from build123d import *

# Parameters (mm, degrees)
SKETCH_R        = 7.5
PAD_DEPTH       = 92
POCKET_DEPTH    = 3
POCKET001_DEPTH = 9.701
POCKET002_DEPTH = 3.7


with BuildPart() as part:
    # Sketch → Pad (new body)
    with BuildSketch(Plane.YZ):
        with BuildLine():
            Line((-25.389858, -4.25), (17.999978, -4.25))
            ThreePointArc((17.999978, -4.25), (22.123115, 11.683029), (10.788897, -0.25))
            Line((-10.788897, -0.25), (10.788897, -0.25))
            ThreePointArc((-10.788897, -0.25), (-13.649082, 11.552021), (-25.389858, 8.45))
            Line((-43.389858, 8.45), (-25.389858, 8.45))
            Line((-43.389858, -4.25), (-43.389858, 8.45))
            Line((-25.389858, -4.25), (-43.389858, -4.25))
        make_face()
        with Locations((-18, 4.25)):
            Circle(SKETCH_R, mode=Mode.SUBTRACT)
        with Locations((18, 4.25)):
            Circle(SKETCH_R, mode=Mode.SUBTRACT)
    extrude(amount=PAD_DEPTH)

    # Sketch001 → Pocket (cut)
    with BuildSketch(Plane(origin=(0, 0, 8.45), x_dir=(0, -1, 0), z_dir=(0, 0, 1))):
        with BuildLine():
            ThreePointArc((43.35, 24), (35.35, 16), (43.35, 8))
            Line((50.35, 8), (43.35, 8))
            Line((50.35, 24), (50.35, 8))
            Line((43.35, 24), (50.35, 24))
        make_face()
        with BuildLine():
            ThreePointArc((43.349998, 84), (35.35, 76), (43.349998, 68))
            Line((59.835098, 68), (43.349998, 68))
            Line((59.835098, 84), (59.835098, 68))
            Line((43.349998, 84), (59.835098, 84))
        make_face()
    extrude(amount=-POCKET_DEPTH, mode=Mode.SUBTRACT)

    # Sketch002 → Pocket001 (cut, through all)
    with BuildSketch(Plane(origin=(0, 0, 5.45), x_dir=(0, -1, 0), z_dir=(0, 0, 1))):
        with BuildLine():
            ThreePointArc((43.35, 22), (37.35, 16), (43.35, 10))
            Line((53.35, 10), (43.35, 10))
            Line((53.35, 22), (53.35, 10))
            Line((43.35, 22), (53.35, 22))
        make_face()
        with BuildLine():
            ThreePointArc((43.35, 82), (37.35, 76.000014), (43.349973, 70))
            Line((53.35, 70), (43.349973, 70))
            Line((53.35, 82), (53.35, 70))
            Line((43.35, 82), (53.35, 82))
        make_face()
    extrude(amount=-POCKET001_DEPTH, mode=Mode.SUBTRACT)

    # Sketch003 → Pocket002 (cut)
    with BuildSketch(Plane.YX.offset(4.25)):
        with BuildLine():
            ThreePointArc((-43.349996, 68), (-35.35, 76.000002), (-43.35, 84))
            Line((-43.35, 84), (-53.35, 84))
            Line((-53.35, 84), (-53.35, 68))
            Line((-53.35, 68), (-43.349996, 68))
        make_face()
        with BuildLine():
            ThreePointArc((-43.35, 8), (-35.35, 16), (-43.35, 24))
            Line((-43.35, 24), (-53.350004, 24))
            Line((-53.350004, 24), (-53.350004, 8))
            Line((-53.350004, 8), (-43.35, 8))
        make_face()
    extrude(amount=-POCKET002_DEPTH, mode=Mode.SUBTRACT)


solid = part.part
Read the model definition and answer for the solid it produces. Units are mm, in the model's axes. A direction names the side the tool comes from. Round coordinates to 2 decimals unless told otherwise and drop trailing zeros. Loops run counter-clockwise (first coordinate to the right, second up) from the corner with the lowest first, then second, coordinate; pieces in that order, holes last.
Q1. Each of these flat-tipped pins is pushed along its axis until it touches: pin 1 (6.5 mm diameter, centred on x = 59, y = -4.5, fed in from +Z); pin 2 (4 mm diameter, centred on x = 80, y = -39.5, fed in from -Z); pin 3 (10 mm diameter, centred on y = 9.5, z = 10.5, fed in from -X); pin 4 (5.5 mm diameter, centred on x = 69, y = -35.5, fed in from +Z). Where does it stop, or does it pass through?
Q2. Section D-D on x = 16 is taken. Write down the section's boundary in (y, z), and give its area (3 significant figures).
Q3. Consider probe 1 along Y at (x, z) = (48, 4); probe 2 along Z at (x, y) = (72, -18); probe 3 along Y at (x, z) = (19, 6.5). Determine where each line is inside the solid, lowest interval first.
Q4. Which of the six approach directions +Z, -Z, +X, -X, +Y, -Y give full straight-line access (tool end or side, diameter ignored) to faces 4 (the face through (45.356, 12.472, 9.319)), 5 (the face through (92, -22, -3)), 6 (the face through (75, -37, -0.55)), 7 (the face through (45, -35, 8.45)), 8 (the face through (76.176, -35.352, 6.971))?
Q5. Section C-C on z = 4.25 is taken. Give the number of separate pieces and of enclosed holes in the cut face, and give its area (3 significant figures).
Q6. Section A-A on y = -18 is taken. Write down the section's boundary in (x, z).
Q7. Section B-B on x = 30 is taken. Write down the section's boundary in (y, z).
Q8. Determine the mould class of faces 1 (the face through (15, -37, -0.55)), 2 (the face through (45.356, -13.487, 11.453)), 3 (the face through (0, -22, -3)) for opening direction Z: released by +Z, released by -Z, zero draft, split by the parting line, or undercut.
Output:
1. pin 1: stops at z = -0.25
1. pin 2: stops at z = -0.55
1. pin 3: stops at x = 0
1. pin 4: stops at z = 8.45
2. outline: (-37.35, -0.55) - (-35.35, -0.55) - (-35.35, -4.25) - (18, -4.25) arc R8.5 ccw (long way) to (10.79, -0.25) - (-10.79, -0.25) arc R8.5 ccw (long way) to (-25.39, 8.45) - (-35.35, 8.45) - (-35.35, 5.45) - (-37.35, 5.45) - close; hole circle Ø15 at (-18, 4.25); hole circle Ø15 at (18, 4.25)
2. area: 345 mm2
3. probe 1: y = -43.39 to -25.5, -10.5 to -9.5, 9.5 to 10.5, 25.5 to 26.5
3. probe 2: z = -4.25 to -3.25, 11.75 to 12.75
3. probe 3: y = -35.93 to -25.15, -10.85 to -9.8, 9.8 to 10.85, 25.15 to 26.2
4. face 4: +X, -X
4. face 5: +Z, -Z, +X, +Y, -Y
4. face 6: -Z, -Y
4. face 7: +Z, +X, -X, -Y
4. face 8: +Z, -Y
5. separate pieces: 4
5. enclosed holes: 0
5. area: 1,810 mm2
6. outline: (0, -4.25) - (92, -4.25) - (92, -3.25) - (0, -3.25) - close; (0, 11.75) - (92, 11.75) - (92, 12.75) - (0, 12.75) - close
7. outline: (-43.39, -4.25) - (18, -4.25) arc R8.5 ccw (long way) to (10.79, -0.25) - (-10.79, -0.25) arc R8.5 ccw (long way) to (-25.39, 8.45) - (-43.39, 8.45) - close; hole circle Ø15 at (-18, 4.25); hole circle Ø15 at (18, 4.25)
8. face 1: released by -Z
8. face 2: undercut
8. face 3: zero draft
